```python
from build123d import *

# Parameters (mm, degrees)
BOSS_EXTRUDE1_DEPTH = 9.1
BOSS_EXTRUDE2_DEPTH = 30.2
BOSS_EXTRUDE3_DEPTH = 8.1
SKETCH4_R           = 15.875
CUT_EXTRUDE1_DEPTH  = 0.7
SKETCH5_R           = 11
BOSS_EXTRUDE4_DEPTH = 2.4
SKETCH6_R           = 1.75
CUT_EXTRUDE2_DEPTH  = 58.200830414
CHAMFER1_SIZE       = 0.5
SKETCH7_R           = 3.95
CUT_EXTRUDE3_DEPTH  = 3.3
SKETCH8_R           = 3.25
CUT_EXTRUDE4_DEPTH  = 5
SKETCH9_R           = 2
BOSS_EXTRUDE5_DEPTH = 27
CHAMFER2_SIZE       = 0.5
SKETCH10_R          = 0.75
CUT_EXTRUDE5_DEPTH  = 3
CHAMFER3_SIZE       = 0.25
SKETCH11_R          = 2.5
BOSS_EXTRUDE6_DEPTH = 0.5
CHAMFER4_SIZE       = 0.5
CUT_EXTRUDE6_START  = -3
SKETCH12_R          = 0.75
CUT_EXTRUDE6_DEPTH  = 3
CHAMFER5_SIZE       = 0.25
SKETCH14_W          = 8
SKETCH14_H          = 7.1
CUT_EXTRUDE8_DEPTH  = 5


with BuildPart() as part:
    # Sketch1 → Boss-Extrude1 (new body)
    with BuildSketch(Plane.XY):
        Polygon((15.75, 20.75), (20.75, 15.75), (20.75, -15.75), (15.75, -20.75), (-15.75, -20.75), (-20.75, -15.75), (-20.75, 15.75), (-15.75, 20.75), align=None)
    extrude(amount=BOSS_EXTRUDE1_DEPTH)

    # Sketch2 → Boss-Extrude2 (add)
    with BuildSketch(Plane.XY.offset(9.1)):
        with BuildLine():
            Line((13.335786438, 20.164213562), (20.164213562, 13.335786438))
            ThreePointArc((20.164213562, 13.335786438), (20.597759065, 12.68693974), (20.75, 11.921572875))
            Line((20.75, 11.921572875), (20.75, -11.921572875))
            ThreePointArc((20.75, -11.921572875), (20.597759065, -12.68693974), (20.164213562, -13.335786438))
            Line((20.164213562, -13.335786438), (13.335786438, -20.164213562))
            ThreePointArc((13.335786438, -20.164213562), (12.68693974, -20.597759065), (11.921572875, -20.75))
            Line((11.921572875, -20.75), (-11.921572875, -20.75))
            ThreePointArc((-11.921572875, -20.75), (-12.68693974, -20.597759065), (-13.335786438, -20.164213562))
            Line((-13.335786438, -20.164213562), (-20.164213562, -13.335786438))
            ThreePointArc((-20.164213562, -13.335786438), (-20.597759065, -12.68693974), (-20.75, -11.921572875))
            Line((-20.75, -11.921572875), (-20.75, 11.921572875))
            ThreePointArc((-20.75, 11.921572875), (-20.597759065, 12.68693974), (-20.164213562, 13.335786438))
            Line((-20.164213562, 13.335786438), (-13.335786438, 20.164213562))
            ThreePointArc((-13.335786438, 20.164213562), (-12.68693974, 20.597759065), (-11.921572875, 20.75))
            Line((-11.921572875, 20.75), (11.921572875, 20.75))
            ThreePointArc((11.921572875, 20.75), (12.68693974, 20.597759065), (13.335786438, 20.164213562))
        make_face()
    extrude(amount=BOSS_EXTRUDE2_DEPTH)

    # Sketch3 → Boss-Extrude3 (add)
    with BuildSketch(Plane.XY.offset(39.3)):
        Polygon((15.75, 20.75), (20.75, 15.75), (20.75, -15.75), (15.75, -20.75), (-15.75, -20.75), (-20.75, -15.75), (-20.75, 15.75), (-15.75, 20.75), align=None)
    extrude(amount=BOSS_EXTRUDE3_DEPTH)

    # Sketch4 → Cut-Extrude1 (cut)
    with BuildSketch(Plane.XY.offset(47.4)):
        Circle(SKETCH4_R)
    extrude(amount=-CUT_EXTRUDE1_DEPTH, mode=Mode.SUBTRACT)

    # Sketch5 → Boss-Extrude4 (add)
    with BuildSketch(Plane.XY.offset(46.7)):
        Circle(SKETCH5_R)
    extrude(amount=BOSS_EXTRUDE4_DEPTH)

    # Sketch6 → Cut-Extrude2 (cut, through all)
    with BuildSketch(Plane(origin=(0, 0, 0), x_dir=(-1, 0, 0), z_dir=(0, 0, -1))):
        with Locations((-15.5, 15.5)):
            Circle(SKETCH6_R)
        with Locations((-15.5, -15.5)):
            Circle(SKETCH6_R)
        with Locations((15.5, -15.5)):
            Circle(SKETCH6_R)
        with Locations((15.5, 15.5)):
            Circle(SKETCH6_R)
    extrude(amount=-CUT_EXTRUDE2_DEPTH, mode=Mode.SUBTRACT)

    # Chamfer1
    chamfer1_edges = [part.edges().sort_by_distance(p)[0] for p in [
        (17.25, 15.5, 47.4),
        (17.25, 15.5, 0),
        (17.25, -15.5, 47.4),
        (17.25, -15.5, 0),
        (-13.75, -15.5, 47.4),
        (-13.75, -15.5, 0),
        (-13.75, 15.5, 47.4),
        (-13.75, 15.5, 0),
    ]]
    chamfer(chamfer1_edges, length=CHAMFER1_SIZE)

    # Sketch7 → Cut-Extrude3 (cut)
    with BuildSketch(Plane(origin=(0, 0, 0), x_dir=(-1, 0, 0), z_dir=(0, 0, -1))):
        Circle(SKETCH7_R)
    extrude(amount=-CUT_EXTRUDE3_DEPTH, mode=Mode.SUBTRACT)

    # Sketch8 → Cut-Extrude4 (cut)
    with BuildSketch(Plane.XY.offset(49.1)):
        Circle(SKETCH8_R)
    extrude(amount=-CUT_EXTRUDE4_DEPTH, mode=Mode.SUBTRACT)

    # Sketch9 → Boss-Extrude5 (add)
    with BuildSketch(Plane.XY.offset(44.1)):
        Circle(SKETCH9_R)
    extrude(amount=BOSS_EXTRUDE5_DEPTH)

    # Chamfer2
    chamfer2_edges = [part.edges().sort_by_distance(p)[0] for p in [
        (-2, 0, 71.1),
    ]]
    chamfer(chamfer2_edges, length=CHAMFER2_SIZE)

    # Sketch10 → Cut-Extrude5 (cut)
    with BuildSketch(Plane.XY.offset(71.1)):
        Circle(SKETCH10_R)
    extrude(amount=-CUT_EXTRUDE5_DEPTH, mode=Mode.SUBTRACT)

    # Chamfer3
    chamfer3_edges = [part.edges().sort_by_distance(p)[0] for p in [
        (-0.75, 0, 71.1),
    ]]
    chamfer(chamfer3_edges, length=CHAMFER3_SIZE)

    # Sketch11 → Boss-Extrude6 (add)
    with BuildSketch(Plane(origin=(0, 0, 3.3), x_dir=(-1, 0, 0), z_dir=(0, 0, -1))):
        Circle(SKETCH11_R)
    extrude(amount=BOSS_EXTRUDE6_DEPTH)

    # Chamfer4
    chamfer4_edges = [part.edges().sort_by_distance(p)[0] for p in [
        (2.5, 0, 2.8),
    ]]
    chamfer(chamfer4_edges, length=CHAMFER4_SIZE - 0.0001)  # a hair under: the kernel refuses the full size

    # Sketch12 → Cut-Extrude6 (cut)
    with BuildSketch(Plane(origin=(0, 0, 2.8), x_dir=(-1, 0, 0), z_dir=(0, 0, -1)).offset(CUT_EXTRUDE6_START)):
        with Locations(Location((0, 0, 0), (0, 0, 180))):
            Circle(SKETCH12_R)
    extrude(amount=CUT_EXTRUDE6_DEPTH, mode=Mode.SUBTRACT)

    # Chamfer5
    chamfer5_edges = [part.edges().sort_by_distance(p)[0] for p in [
        (-0.75, 0, 2.8),
    ]]
    chamfer(chamfer5_edges, length=CHAMFER5_SIZE)

    # Sketch14 → Cut-Extrude8 (cut)
    with BuildSketch(Plane.XZ.offset(20.75)):
        with Locations((0, 4.55)):
            Rectangle(SKETCH14_W, SKETCH14_H)
    extrude(amount=-CUT_EXTRUDE8_DEPTH, mode=Mode.SUBTRACT)


solid = part.part
```
Part model, mm, in its own coordinate system. A direction names the side the tool comes from. Round coordinates to 2 decimals unless told otherwise and drop trailing zeros. Write each loop counter-clockwise with the first axis right and the second up, starting at its lowest first coordinate (ties: lowest second). Pieces come first, ordered by that corner, then holes.
Item 1: Cut at B-B, the plane y = 9.5. Give the cut face in (x, z).
Results:
outline: (-20.75, 0) - (20.75, 0) - (20.75, 47.4) - (12.72, 47.4) - (12.72, 46.7) - (5.55, 46.7) - (5.55, 49.1) - (-5.55, 49.1) - (-5.55, 46.7) - (-12.72, 46.7) - (-12.72, 47.4) - (-20.75, 47.4) - close
Item 2: Cut at A-A, the plane z = 29.5. Give the cut face in (x, y), plus the area to 3 significant figures.
Results:
outline: (-20.75, -11.92) arc R2 ccw to (-20.16, -13.34) - (-13.34, -20.16) arc R2 ccw to (-11.92, -20.75) - (11.92, -20.75) arc R2 ccw to (13.34, -20.16) - (20.16, -13.34) arc R2 ccw to (20.75, -11.92) - (20.75, 11.92) arc R2 ccw to (20.16, 13.34) - (13.34, 20.16) arc R2 ccw to (11.92, 20.75) - (-11.92, 20.75) arc R2 ccw to (-13.34, 20.16) - (-20.16, 13.34) arc R2 ccw to (-20.75, 11.92) - close; hole circle Ø3.5 at (-15.5, -15.5); hole circle Ø3.5 at (-15.5, 15.5); hole circle Ø3.5 at (15.5, -15.5); hole circle Ø3.5 at (15.5, 15.5)
area: 1,560 mm2
Item 3: Probe L1, parallel to Y at x = 0, z = 46.05; L2, parallel to Y at x = 0, z = 47.15 (3 decimals); L3, parallel to Y at x = -15, z = 12. List the from-to ranges inside material, lowest first.
Results:
L1: y = -20.75 to -3.25, -2 to 2, 3.25 to 20.75
L2: y = -20.75 to -15.875, -11 to -3.25, -2 to 2, 3.25 to 11, 15.875 to 20.75
L3: y = -18.5 to -17.18, -13.82 to 13.82, 17.18 to 18.5
Item 4: Cut at D-D, the plane x = 6. Give the cut face in (y, z).
Results:
outline: (-20.75, 0) - (20.75, 0) - (20.75, 47.4) - (14.7, 47.4) - (14.7, 46.7) - (9.22, 46.7) - (9.22, 49.1) - (-9.22, 49.1) - (-9.22, 46.7) - (-14.7, 46.7) - (-14.7, 47.4) - (-20.75, 47.4) - close
Item 5: Two-plate mould, pull along Y, no slides. Class faces 1 (the cylindrical face through (-0.75, 0.03, 69.49)), 2 (the flat face through (-3, -2, 49.1)), 3 (the flat face through (0, -15.75, 5)): +Y half, -Y half, draft (parallel to the pull), parting line (faces both ways), or undercut.
Results:
face 1: undercut
face 2: draft
face 3: -Y half
Item 6: Cut at C-C, the plane z = 42. Give the cut face in (x, y).
Results:
outline: (-20.75, -15.75) - (-15.75, -20.75) - (15.75, -20.75) - (20.75, -15.75) - (20.75, 15.75) - (15.75, 20.75) - (-15.75, 20.75) - (-20.75, 15.75) - close; hole circle Ø3.5 at (-15.5, -15.5); hole circle Ø3.5 at (-15.5, 15.5); hole circle Ø3.5 at (15.5, -15.5); hole circle Ø3.5 at (15.5, 15.5)
Item 7: Which spindle directions (+Z, -Z, +X, -X, +Y, -Y) get a long thin tool onto all of the face, cutting with end or side? Do faces 4 (the flat face through (1, -2, 44.1)), 5 (the cylindrical face through (0.715, -0.225, 4.444)), 6 (the flat face through (-17, -17, 39.3)), 7 (the cylindrical face through (12.697, -20.594, 23.989)), 8 (the flat face through (17, 18, 9.1)). Say none if no direction does.
Results:
face 4: +Z
face 5: -Z
face 6: -X, -Y
face 7: +X, -Y
face 8: +X, +Y
Item 8: Drop flat-ended pins along their axis: pin 1 Ø5.5 at (x, y) = (-0.5, -19) entering from -Z; pin 2 Ø2 at (x, y) = (15.5, 15.5) entering from -Z; pin 3 Ø1.5 at (y, z) = (-18, 5.5) entering from -X; pin 4 Ø5.5 at (x, y) = (-15.5, -15.5) entering from +Z. Give the stop position or say it passes through.
Results:
pin 1: stops at z = 0
pin 2: passes through
pin 3: stops at x = -19.25
pin 4: stops at z = 47.4
